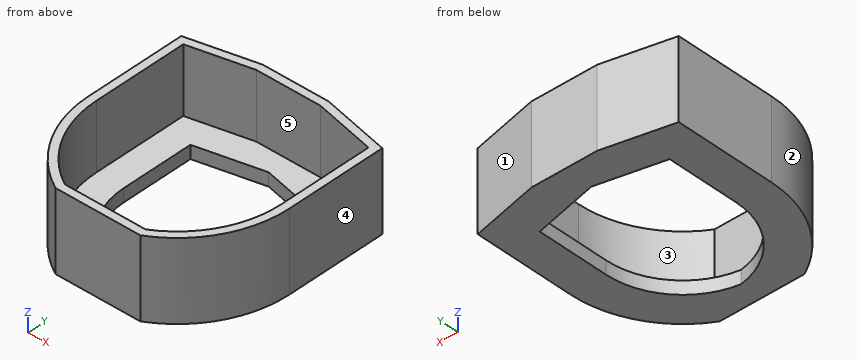
```python
from build123d import *

# Parameters (mm, degrees)
F2_DEPTH = 12.7
F4_DEPTH = 2.54
F5_DEPTH = 25.4


with BuildPart() as f2:
    # F1 (on Top) → F2 (new body)
    with BuildSketch(Plane.XY):
        with BuildLine():
            Line((6.339406, 21.194164), (-6.339406, 21.194164))
            Line((-6.339406, 21.194164), (-19.3675, 18.299032))
            Line((-19.3675, 18.299032), (-19.3675, -1.016))
            ThreePointArc((-19.3675, -1.016), (-16.359844, -12.015319), (-8.173823, -19.953836))
            Line((-8.173823, -19.953836), (8.173823, -19.953836))
            ThreePointArc((8.173823, -19.953836), (16.359844, -12.015319), (19.3675, -1.016))
            Line((19.3675, -1.016), (19.3675, 18.299032))
            Line((19.3675, 18.299032), (6.339406, 21.194164))
        make_face()
        with BuildLine():
            Line((7.774487, -18.429836), (-7.774487, -18.429836))
            ThreePointArc((-7.774487, -18.429836), (-15.145045, -11.073668), (-17.8435, -1.016))
            Line((-17.8435, -1.016), (-17.8435, 17.076522))
            Line((-17.8435, 17.076522), (-6.172113, 19.670164))
            Line((-6.172113, 19.670164), (6.172113, 19.670164))
            Line((6.172113, 19.670164), (17.8435, 17.076522))
            Line((17.8435, 17.076522), (17.8435, -1.016))
            ThreePointArc((17.8435, -1.016), (15.145045, -11.073668), (7.774487, -18.429836))
        make_face(mode=Mode.SUBTRACT)
    extrude(amount=F2_DEPTH)

    # F3 (on face) → F4 (join)
    with BuildSketch(Plane(origin=(0, 0, 0), x_dir=(1, 0, 0), z_dir=(0, 0, -1))):
        with BuildLine():
            Line((8.173823, 19.953836), (-8.173823, 19.953836))
            ThreePointArc((-8.173823, 19.953836), (-16.359844, 12.015319), (-19.3675, 1.016))
            Line((-19.3675, 1.016), (-19.3675, -18.299032))
            Line((-19.3675, -18.299032), (-6.339406, -21.194164))
            Line((-6.339406, -21.194164), (6.339406, -21.194164))
            Line((6.339406, -21.194164), (19.3675, -18.299032))
            Line((19.3675, -18.299032), (19.3675, 1.016))
            ThreePointArc((19.3675, 1.016), (16.359844, 12.015319), (8.173823, 19.953836))
        make_face()
    extrude(amount=F4_DEPTH)

    # F1 (on Top) → F5 (cut)
    with BuildSketch(Plane.XY):
        with BuildLine():
            Line((12.5095, 12.797739), (0, 15.577628))
            Line((0, 15.577628), (-12.5095, 12.797739))
            Line((-12.5095, 12.797739), (-12.5095, -1.016))
            ThreePointArc((-12.5095, -1.016), (-8.953801, -10.623903), (0, -15.60228))
            ThreePointArc((0, -15.60228), (8.953801, -10.623903), (12.5095, -1.016))
            Line((12.5095, -1.016), (12.5095, 12.797739))
        make_face()
    extrude(amount=-F5_DEPTH, mode=Mode.SUBTRACT)


solid = f2.part
```
Here's how the part is built. I have some questions about the finished solid (model axes, mm). Face numbers are marked on the shaded views. A direction names the side the tool comes from. Round coordinates to 2 decimals unless told otherwise and drop trailing zeros. Order: outer loops, then holes, each group sorted by start corner. A loop starts at its lowest first (then second) coordinate and runs counter-clockwise, first axis right, second up. Notation, with made-up numbers: M 33.5,49.5 L 37.5,49.5 A30 ccw 37.5,83.5 Z; hole C 13.5,27.25 d11. An arc over 180 degrees is marked long. One line per question, with ' | ' between items.
1) I need wall thicknesses on line 1 along Y through (x, z) = (5, 7.5); line 2 along X through (y, z) = (7, 1); line 3 along X through (y, z) = (2.5, -1.25). Which ranges of each line are inside material? Lowest first, please.
Working result:
line 1: -19.95 to -18.43, 19.67 to 21.19 | line 2: -19.37 to -17.84, 17.84 to 19.37 | line 3: -19.37 to -12.51, 12.51 to 19.37
2) If we mould it in two halves opening along Y, with no side actions, what happens to the marked faces 1, 2 and 3? For each: +Y half, -Y half, draft (parallel to the pull), parting line (faces both ways), or undercut.
Working result:
face 1: +Y half | face 2: -Y half | face 3: undercut
3) I want a section at B-B, the plane z = 11.5. Write out the boundary of the cut face in (x, y), then the cut area to 3 significant figures.
Working result:
outline: M -19.37,-1.02 A21.62 ccw -8.17,-19.95 L 8.17,-19.95 A21.62 ccw 19.37,-1.02 L 19.37,18.3 L 6.34,21.19 L -6.34,21.19 L -19.37,18.3 Z; hole M -17.84,-1.02 A20.09 ccw -7.77,-18.43 L 7.77,-18.43 A20.09 ccw 17.84,-1.02 L 17.84,17.08 L 6.17,19.67 L -6.17,19.67 L -17.84,17.08 Z | area: 206 mm²
4) I want a section at A-A, the plane y = 0.5. Write out the boundary of the cut face in (x, z), then the cut area to 3 significant figures.
Working result:
outline: M -19.37,-2.54 L -12.51,-2.54 L -12.51,0 L -17.84,0 L -17.84,12.7 L -19.37,12.7 Z; M 12.51,-2.54 L 19.37,-2.54 L 19.37,12.7 L 17.84,12.7 L 17.84,0 L 12.51,0 Z | area: 73.5 mm²
5) I want a section at C-C, the plane x = 4.5. Write out the boundary of the cut face in (y, z).
Working result:
outline: M -19.95,-2.54 L -14.14,-2.54 L -14.14,0 L -18.43,0 L -18.43,12.7 L -19.95,12.7 Z; M 14.58,-2.54 L 21.19,-2.54 L 21.19,12.7 L 19.67,12.7 L 19.67,0 L 14.58,0 Z
6) I want a section at D-D, the plane x = 14.5. Write out the boundary of the cut face in (y, z), then the cut area to 3 significant figures.
Working result:
outline: M -14.68,-2.54 L 19.38,-2.54 L 19.38,12.7 L 17.82,12.7 L 17.82,0 L -12.11,0 L -12.11,12.7 L -14.68,12.7 Z | area: 139 mm²
7) For pin 1 Ø4 at (x, y) = (-3, 14.5) entering from +Z; pin 2 Ø3 at (x, z) = (-14, 8.5) entering from -Y; pin 3 Ø3 at (x, y) = (5.5, -11.5) entering from -Z; pin 4 Ø1 at (y, z) = (-8, 4.5) entering from +X, each with a flat end and sliding along its axis, tell me the tip position at first contact or that it passes through.
Working result:
pin 1: z = 0 | pin 2: y = -16.82 | pin 3: through | pin 4: x = 18.37
8) For the marked faces 4 and 5, which set-ups out of +Z, -Z, +X, -X, +Y, -Y let a thin tool reach every point of the face, with its end or its side?
Working result:
face 4: +Z, -Z, +X, +Y, -Y | face 5: +Z
